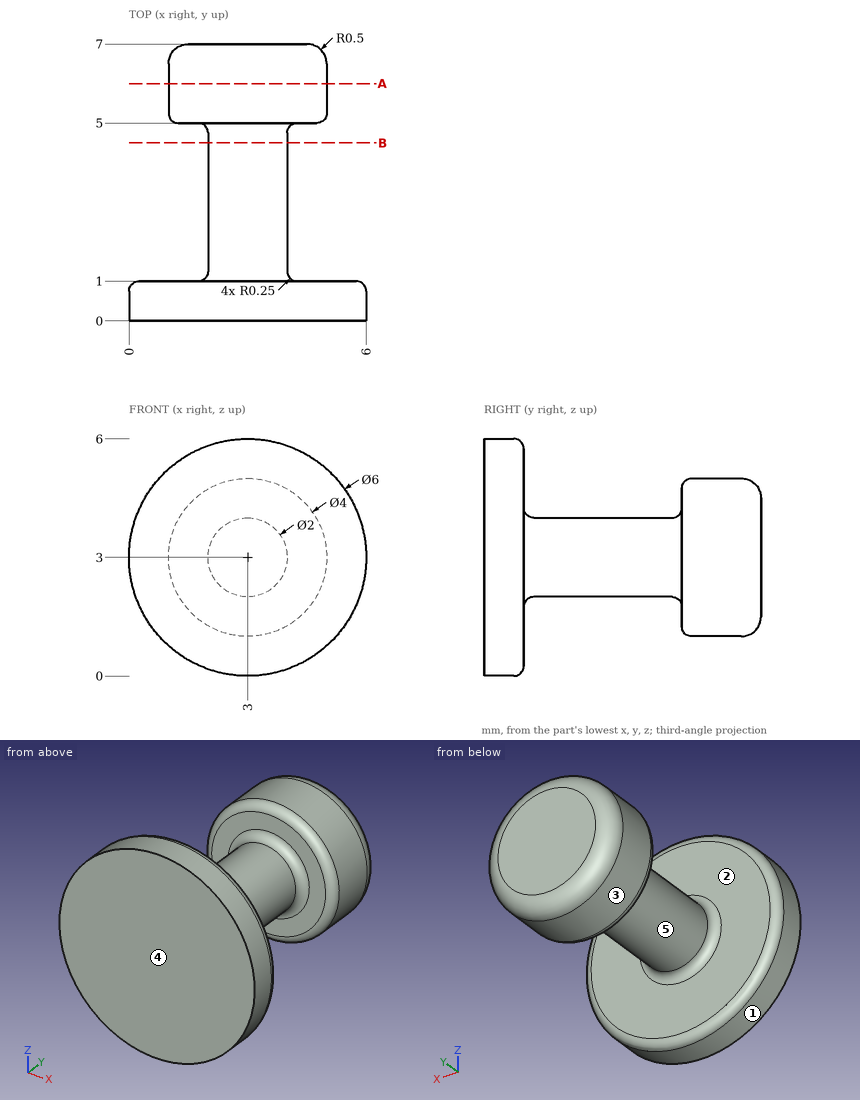
Answer from the drawing. Dimensions are ordinates in mm from the lowest x, y and z of the part. A direction names the side the tool comes from. Give positions to 0.01 mm unless a question says otherwise; leave off trailing zeros. Write each loop counter-clockwise with the first axis right and the second up, starting at its lowest first coordinate (ties: lowest second). Pieces come first, ordered by that corner, then holes.
1) Section A-A (y = 6) is taken. Write down the section's boundary in (x, z).
2) A tool of negligible diameter and unlimited length cuts with its end or side. For the marked faces 1 and 2, from which of +Z, -Z, +X, -X, +Y, -Y can it reach the whole face along a straight path? Write none if from no direction.
3) Find the intervals of material crossed by L1, parallel to Y at x = 4.5, z = 3; L2, parallel to Y at x = 1, z = 3.5; L3, parallel to Y at x = 3.75, z = 3.75, in increasing order.
4) For a pull along Y with two mould halves and no side action, classify the marked faces 3, 4 and 5 as pulls with the +Y half, pulls with the -Y half, needs draft (parallel to the pull), parting line crosses it, or undercut.
5) Section B-B (y = 4.5) is taken. Write down the section's boundary in (x, z), and give its area (3 significant figures).
Response:
1. outline: circle Ø4 at (3, 3)
2. face 1: +Y, -Y
2. face 2: none
3. L1: y = 0 to 1, 5 to 7
3. L2: y = 0 to 1
3. L3: y = 0 to 1.09, 4.91 to 7
4. face 3: needs draft
4. face 4: pulls with the -Y half
4. face 5: undercut
5. outline: circle Ø2 at (3, 3)
5. area: 3.14 mm2
